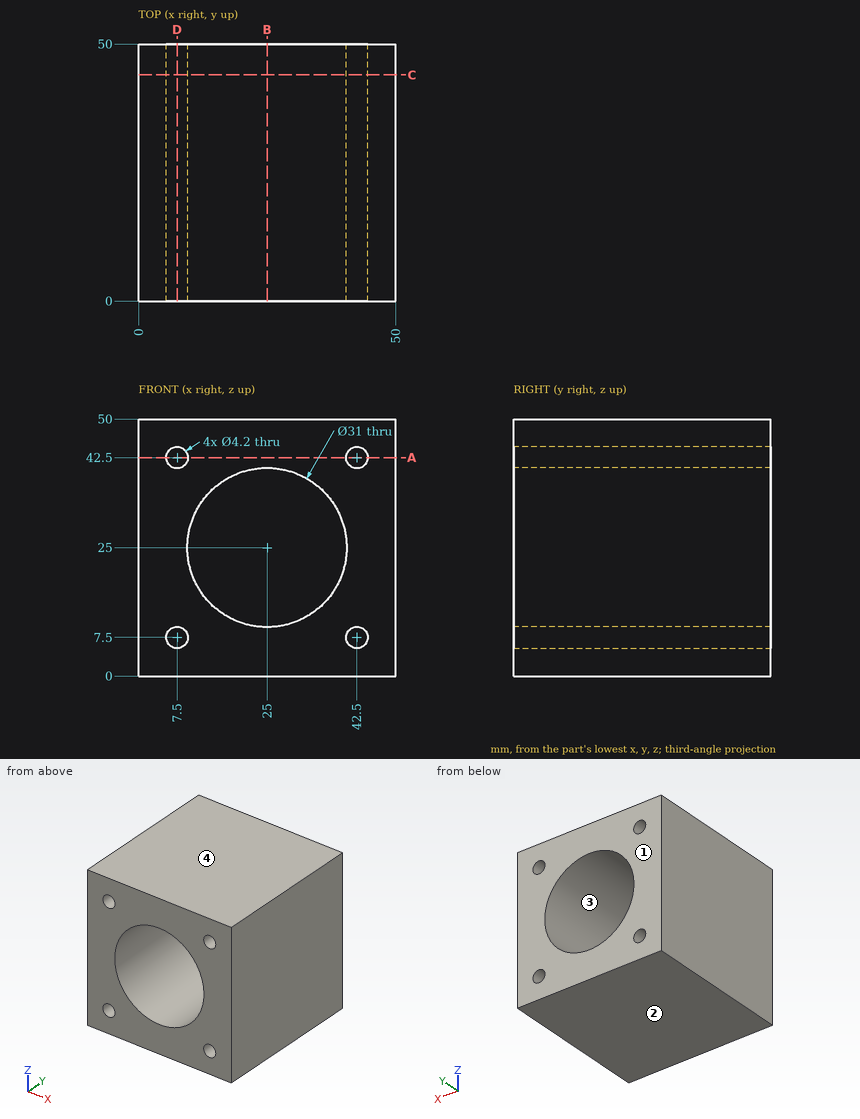
Part print with two shaded views. Sizes in mm from the minimum x, y, z corner. Round coordinates to 2 decimals unless told otherwise and drop trailing zeros. Order: outer loops, then holes, each group sorted by start corner. A loop starts at its lowest first (then second) coordinate and runs counter-clockwise, first axis right, second up. Notation, with made-up numbers: (81.25, 37.5) - (104.25, 37.5) arc R27 ccw to (104.25, 59.5) - close; hole circle Ø6 at (-22, 5). An arc over 180 degrees is marked (long way). Answer in a Markdown table with one row per item. Add a question column.
(1) Band-saw the part on B-B on x = 25. List the corners of the cut face in (y, z).
(2) Band-saw the part on D-D on x = 7.5. List the corners of the cut face in (y, z), and give its area (3 significant figures).
(3) Drop flat-ended pins along their axis: pin 1 Ø5.5 at (x, z) = (7.5, 42.5) entering from -Y; pin 2 Ø4 at (x, z) = (7.5, 7.5) entering from +Y. Give the stop position or say it passes through.
(4) Band-saw the part on C-C on y = 44. List the corners of the cut face in (x, z), and give its area (3 significant figures).
(5) Band-saw the part on A-A on z = 42.5. List the corners of the cut face in (x, y).
(6) Probe L1, parallel to X at y = 11, z = 7.5; L2, parallel to X at y = 9.5, z = 6; L3, parallel to X at y = 24.5, z = 25. List the from-to ranges inside material, lowest first. Write a range as [from, to].
(7) Mould opens along Z. For the marked faces 1, 2, 3 and 4 say: +Z half, -Z half, draft (parallel to the pull), parting line (faces both ways), or undercut.
Data:
| question | item | result |
|---|---|---|
| 1 | outline | (0, 0) - (50, 0) - (50, 9.5) - (0, 9.5) - close; (0, 40.5) - (50, 40.5) - (50, 50) - (0, 50) - close |
| 2 | outline | (0, 0) - (50, 0) - (50, 5.4) - (0, 5.4) - close; (0, 9.6) - (50, 9.6) - (50, 40.4) - (0, 40.4) - close; (0, 44.6) - (50, 44.6) - (50, 50) - (0, 50) - close |
| 2 | area | 2,080 mm^2 |
| 3 | pin 1 | stops at y = 0 |
| 3 | pin 2 | passes through |
| 4 | outline | (0, 0) - (50, 0) - (50, 50) - (0, 50) - close; hole circle Ø4.2 at (7.5, 7.5); hole circle Ø4.2 at (7.5, 42.5); hole circle Ø31 at (25, 25); hole circle Ø4.2 at (42.5, 7.5); hole circle Ø4.2 at (42.5, 42.5) |
| 4 | area | 1,690 mm^2 |
| 5 | outline | (0, 0) - (5.4, 0) - (5.4, 50) - (0, 50) - close; (9.6, 0) - (40.4, 0) - (40.4, 50) - (9.6, 50) - close; (44.6, 0) - (50, 0) - (50, 50) - (44.6, 50) - close |
| 6 | L1 | x = [0, 5.4], [9.6, 40.4], [44.6, 50] |
| 6 | L2 | x = [0, 6.03], [8.97, 41.03], [43.97, 50] |
| 6 | L3 | x = [0, 9.5], [40.5, 50] |
| 7 | face 1 | draft |
| 7 | face 2 | -Z half |
| 7 | face 3 | undercut |
| 7 | face 4 | +Z half |
